Read the model definition and answer for the solid it produces. Units are mm, in the model's axes. A direction names the side the tool comes from. Round coordinates to 2 decimals unless told otherwise and drop trailing zeros. Write each loop counter-clockwise with the first axis right and the second up, starting at its lowest first coordinate (ties: lowest second). Pieces come first, ordered by that corner, then holes. Notation, with made-up numbers: (31.5, 80) - (75.5, 80) arc R11 ccw to (75.5, 97) - close; hole circle Ø6 at (-36.5, 12). An arc over 180 degrees is marked (long way). Answer as CSV lines item,"result". Start each with the question number.
1) Consider line 1 along X through (y, z) = (14.5, 39.5); line 2 along Y through (x, z) = (27.5, -26.5). Determine where each line is inside the solid, lowest interval first.
2) Find section A-A on z = 32.5. Determine the outline of the cut face in (x, y), then the cut area to 3 significant figures.
3) Each of these flat-tipped pins is pushed along its axis until it touches: pin 1 (3 mm diameter, centred on y = 15.5, z = 0.5, fed in from +X); pin 2 (10 mm diameter, centred on x = -33, z = 8, fed in from +Y). Where does it stop, or does it pass through?
4) Find section C-C on y = 11.25. Determine the outline of the cut face in (x, z), then the cut area to 3 significant figures.
5) Find section B-B on x = 36. Determine the outline of the cut face in (y, z), then the cut area to 3 significant figures.
6) Which of the six approach directions +Z, -Z, +X, -X, +Y, -Y give full straight-line access (tool end or side, diameter ignored) to faces 1 (the flat face through (-1, 8, -50)), 2 (the flat face through (21.5, 15, -1)), 3 (the flat face through (-33, 10, -1))?
from build123d import *

# Parameters (mm, degrees)
SKETCH_1_W      = 89
SKETCH_1_H      = 100
EXTRUDE_1_DEPTH = 10
EXTRUDE_2_DEPTH = 10


with BuildPart() as part:
    # Эскиз1 → Бобышка-Вытянуть1 (new body)
    with BuildSketch(Plane(origin=(0, 0, 0), x_dir=(1, 0, 0), z_dir=(0, 1, 0))):
        Rectangle(SKETCH_1_W, SKETCH_1_H)
    extrude(amount=EXTRUDE_1_DEPTH)

    # Эскиз2 → Бобышка-Вытянуть2 (add)
    with BuildSketch(Plane(origin=(0, 10, 0), x_dir=(1, 0, 0), z_dir=(0, 1, 0))):
        Polygon((0, 50), (21.5, 50), (21.5, -50), (-21.5, -50), (-21.5, 50), align=None)
    extrude(amount=EXTRUDE_2_DEPTH)


solid = part.part
Check values:
1,line 1,"x = -21.5 to 21.5"
1,line 2,"y = 0 to 10"
2,outline,"(-44.5, 0) - (44.5, 0) - (44.5, 10) - (21.5, 10) - (21.5, 20) - (-21.5, 20) - (-21.5, 10) - (-44.5, 10) - close"
2,area,"1,320 mm^2"
3,pin 1,"stops at x = 21.5"
3,pin 2,"stops at y = 10"
4,outline,"(-21.5, -50) - (21.5, -50) - (21.5, 50) - (-21.5, 50) - close"
4,area,"4,300 mm^2"
5,outline,"(0, -50) - (10, -50) - (10, 50) - (0, 50) - close"
5,area,"1,000 mm^2"
6,face 1,"-Z, +X, -X, +Y, -Y"
6,face 2,"+Z, -Z, +X, +Y"
6,face 3,"+Z, -Z, -X, +Y"
